Work out the finished part from the listing and answer in its coordinate system (mm). Coordinates: 2 decimals unless noted, no trailing zeros. Order: outer loops, then holes, each group sorted by start corner. A loop starts at its lowest first (then second) coordinate and runs counter-clockwise, first axis right, second up.
1. Find the intervals of material crossed by probe 1 along Y at (x, z) = (-13.5, 8.5); probe 2 along X at (y, z) = (8.5, 10.75); probe 3 along X at (y, z) = (0, 11.5), in increasing order.
2. Determine the mould class of faces 1 (the cylindrical face through (0, 2, 8)), 2 (the cylindrical face through (2.331, 15.744, 7.395)), 3 (the cylindrical face through (14.253, -7.082, 7.395)) for opening direction Y: +Y half, -Y half, draft (parallel to the pull), parting line (faces both ways), or undercut.
3. The part is cut by section A-A, the plane y = 7. Give the vertices of the cut face in (x, z), then the cut area to 3 significant figures.
4. Flat-ended cylindrical pins translate along their axes: pin 1 Ø6 at (y, z) = (5.5, 3) entering from +X; pin 2 Ø3 at (x, z) = (-3, 10.5) entering from -Y; pin 3 Ø8 at (y, z) = (10.5, 7) entering from -X. Find the tip coordinate at first contact, or state that the pin passes through.
```python
from build123d import *

# Parameters (mm, degrees)
SKETCH_1_R               = 15.91549431
EXTRUDE_1_DEPTH          = 15
CUT_EXTRUDE_1_DEPTH      = 15
SKETCH_3_RX              = 2
SKETCH_3_RY              = 1
CUT_EXTRUDE_2_DEPTH      = 15
PATTERN_CIRCULAR_1_COUNT = 20


with BuildPart() as part:
    # Эскиз1 → Бобышка-Вытянуть1 (new body)
    with BuildSketch(Plane.XY):
        Circle(SKETCH_1_R)
    extrude(amount=EXTRUDE_1_DEPTH)

    # Эскиз2 → Вырез-Вытянуть1 (cut)
    with BuildSketch(Plane.XY.offset(15)):
        with BuildLine():
            Line((-1.475635456, -1.35), (1.475635456, -1.35))
            ThreePointArc((1.475635456, -1.35), (0, 2), (-1.475635456, -1.35))
        make_face()
    extrude(amount=-CUT_EXTRUDE_1_DEPTH, mode=Mode.SUBTRACT)

    # Эскиз3 → Вырез-Вытянуть2 (cut)
    with BuildSketch(Plane.XY.offset(15)):
        with Locations(Location((12.768681862, 9.500722217), (0, 0, 34.851328061))):
            Ellipse(SKETCH_3_RX, SKETCH_3_RY)
    cut_extrude_2 = extrude(amount=-CUT_EXTRUDE_2_DEPTH, mode=Mode.SUBTRACT)

    # Круговой массив1: Вырез-Вытянуть2 ×20 about axis
    pattern_circular_1_axis = Axis((0, 0, 15), (0, 0, 1))
    for i in range(1, PATTERN_CIRCULAR_1_COUNT):
        add(cut_extrude_2.rotate(pattern_circular_1_axis, i * 360 / PATTERN_CIRCULAR_1_COUNT), mode=Mode.SUBTRACT)


solid = part.part
```
Geometry says:
1. probe 1: y = -8.43 to -5.34, -4.14 to 3.83, 4.81 to 8.35
1. probe 2: x = -11.29 to 11.06, 13.06 to 13.46
1. probe 3: x = -13.96 to -2, 2 to 13.96
2. face 1: undercut
2. face 2: +Y half
2. face 3: -Y half
3. outline: (-14.29, 0) - (14.29, 0) - (14.29, 15) - (-14.29, 15) - close
3. area: 429 mm2
4. pin 1: stops at x = 15.72
4. pin 2: stops at y = -15.84
4. pin 3: stops at x = -14.53
